Source: CAD feature listing. Evaluate the final solid. Frame: model axes, mm. A direction names the side the tool comes from. Give positions to 0.01 mm unless a question says otherwise; leave off trailing zeros. Order: outer loops, then holes, each group sorted by start corner. A loop starts at its lowest first (then second) coordinate and runs counter-clockwise, first axis right, second up. Notation, with made-up numbers: M 60,66.5 L 118,66.5 A29 ccw 118,90.5 Z; hole C 84.25,-25 d10. An arc over 180 degrees is marked long. Use CSV: the item, a comma, the result in double quotes. Start each with the question number.
Item 1: Section query A-A on x = 0. Return loops of the section in (y, z).
Item 2: First-contact query: pin 1 (3 mm diameter, centred on x = -10, y = -2, fed in from +Z). Flat tip, straight axial feed; report the tip coordinate or a pass-through.
Item 3: Access query for faces 3 (the face through (-14, 3.15, 59)), 4 (the face through (-3.15, 14, 59)), 5 (the face through (-4, -12.5, 59)). Directions: +Z, -Z, +X, -X, +Y, -Y. A direction counts if a zero-diameter tool reaches every point of the face in a straight line with its end or side. Return the directions, or none.
Item 4: Section query B-B on y = 10. Return loops of the section in (x, z), and give its area (3 significant figures).
Item 5: Ray query, probe 1 along Y at (x, z) = (9.75, 9); probe 2 along Y at (x, z) = (-3.5, 85); probe 3 along Y at (x, z) = (13.75, 60). Return the intervals inside material, ascending. Write a range as from..to.
Item 6: Pull-direction query (X, two-part tool) for faces 1 (the face through (9, -15, 59)), 2 (the face through (12.77, 8.85, 59.16)); classes: +X half, -X half, draft (parallel to the pull), parting line (faces both ways), or undercut.
from build123d import *

# Parameters (mm, degrees)
F0_R     = 3
F0_R_2   = 2.5
F1_DEPTH = 120


with BuildPart() as f1:
    # F0 (on Top) → F1 (new body)
    with BuildSketch(Plane.XY):
        with BuildLine():
            Line((-15, 15), (-15, 3.15))
            Line((-15, 3.15), (-12.5, 3.15))
            Line((-12.5, 3.15), (-12.5, 5.15))
            Line((-12.5, 5.15), (-6.547707, 5.15))
            ThreePointArc((-6.547707, 5.15), (-4.5, 0), (-6.547707, -5.15))
            Line((-6.547707, -5.15), (-12.5, -5.15))
            Line((-12.5, -5.15), (-12.5, -3.15))
            Line((-12.5, -3.15), (-15, -3.15))
            Line((-15, -3.15), (-15, -15))
            Line((-15, -15), (-3.15, -15))
            Line((-3.15, -15), (-3.15, -12.5))
            Line((-3.15, -12.5), (-5.15, -12.5))
            Line((-5.15, -12.5), (-5.15, -6.547707))
            ThreePointArc((-5.15, -6.547707), (0, -4.5), (5.15, -6.547707))
            Line((5.15, -6.547707), (5.15, -12.5))
            Line((5.15, -12.5), (3.15, -12.5))
            Line((3.15, -12.5), (3.15, -15))
            Line((3.15, -15), (15, -15))
            Line((15, -15), (15, -3.15))
            Line((15, -3.15), (12.5, -3.15))
            Line((12.5, -3.15), (12.5, -5.15))
            Line((12.5, -5.15), (6.547707, -5.15))
            ThreePointArc((6.547707, -5.15), (4.5, 0), (6.547707, 5.15))
            Line((6.547707, 5.15), (12.5, 5.15))
            Line((12.5, 5.15), (12.5, 3.15))
            Line((12.5, 3.15), (15, 3.15))
            Line((15, 3.15), (15, 15))
            Line((15, 15), (3.15, 15))
            Line((3.15, 15), (3.15, 12.5))
            Line((3.15, 12.5), (5.15, 12.5))
            Line((5.15, 12.5), (5.15, 6.547707))
            ThreePointArc((5.15, 6.547707), (0, 4.5), (-5.15, 6.547707))
            Line((-5.15, 6.547707), (-5.15, 12.5))
            Line((-5.15, 12.5), (-3.15, 12.5))
            Line((-3.15, 12.5), (-3.15, 15))
            Line((-3.15, 15), (-15, 15))
        make_face()
        with Locations((-10, -10)):
            Circle(F0_R, mode=Mode.SUBTRACT)
        with Locations((10, -10)):
            Circle(F0_R, mode=Mode.SUBTRACT)
        with Locations((-10, 10)):
            Circle(F0_R, mode=Mode.SUBTRACT)
        Circle(F0_R_2, mode=Mode.SUBTRACT)
        with Locations((10, 10)):
            Circle(F0_R, mode=Mode.SUBTRACT)
    extrude(amount=F1_DEPTH)


solid = f1.part
Verdict:
1,outline,"M -4.5,0 L -2.5,0 L -2.5,120 L -4.5,120 Z; M 2.5,0 L 4.5,0 L 4.5,120 L 2.5,120 Z"
2,pin 1,"through"
3,face 3,"+Z, -Z, -X"
3,face 4,"+Z, -Z, +Y"
3,face 5,"+Z, -Z"
4,outline,"M -15,0 L -13,0 L -13,120 L -15,120 Z; M -7,0 L -5.15,0 L -5.15,120 L -7,120 Z; M 5.15,0 L 7,0 L 7,120 L 5.15,120 Z; M 13,0 L 15,0 L 15,120 L 13,120 Z"
4,area,"924 mm2"
5,probe 1,"-15..-12.99, -7.01..-5.15, 5.15..7.01, 12.99..15"
5,probe 2,"-15..-12.5, -5.37..5.37, 12.5..15"
5,probe 3,"-15..-3.15, 3.15..15"
6,face 1,"draft"
6,face 2,"undercut"
